Geometry: final body of the model. Coordinates: model frame, mm. Round coordinates to 2 decimals unless told otherwise and drop trailing zeros. Write each loop counter-clockwise with the first axis right and the second up, starting at its lowest first coordinate (ties: lowest second). Pieces come first, ordered by that corner, then holes. Notation, with made-up numbers: (16, 40.5) -> (70, 40.5) arc R33 cw to (70, 74.5) -> close; hole circle Ø6 at (40, 1.25). An arc over 180 degrees is marked (long way). Use one line per item in the form item = value. Start each with the question number.
1. Cut plane B-B, the plane y = -3.5. Return the cut outline in (x, z).
2. Pin query (flat end, axial travel): pin 1 Ø4 at (x, y) = (-7.5, 6.5) entering from -Z; pin 2 Ø9 at (x, y) = (0, 0) entering from -Z; pin 3 Ø2 at (x, y) = (8.5, 12.5) entering from -Z; pin 4 Ø5 at (y, z) = (-4, -10.5) entering from +X. Return the tip coordinate at first contact, or that it passes through.
3. Line query: L1, parallel to Y at x = 0, z = 23.2; L2, parallel to Z at x = -7, y = -2.5; L3, parallel to Z at x = 14.5, y = -9. Output: solid intervals per line, ascending.
4. Cut plane C-C, the plane y = 7. Return the cut outline in (x, z), plus the area to 3 significant figures.
5. Draft query along X for faces 1 (the face through (-4, 3, -23)), 2 (the face through (-5.2, -0.27, -23.43)), 3 (the face through (5.1, -19.5, -22.6)), 4 (the face through (-4, -3, 23)). Return one class per face: pulls with the +X half, pulls with the -X half, needs draft (parallel to the pull), parting line crosses it, or undercut.
6. Cut plane D-D, the plane y = 3. Return the cut outline in (x, z).
7. Cut plane A-A, the plane x = 0. Return the cut outline in (y, z).
Autodesk Inventor part; units mm, degrees
ref_plane "YZ Plane" through (0, 0, 0) normal (1, 0, 0) x (0, 1, 0)
ref_plane "XZ Plane" through (0, 0, 0) normal (0, 1, 0) x (-1, 0, 0)
ref_plane "XY Plane" through (0, 0, 0) normal (0, 0, 1) x (1, 0, 0)
sketch "Эскиз1" plane through (0, 0, 0) normal (0, 0, 1) x (1, 0, 0)
  line L0 (0, 19.5) -> (0, -19.5)
  line L1 (23, -19.5) -> (23, 19.5)
  line L2 (23, 19.5) -> (23.6, 19.5)
  line L3 (24, 19.1) -> (24, -19.1)
  line L4 (23.6, -19.5) -> (23, -19.5)
  line L5 (24, -19.1) -> (23.6, -19.5)
  line L6 (24, 19.1) -> (23.6, 19.5)
  point P0 (0, 0)
  point P1 (0, 0)
  point P2 (24, 19.5)
  point P3 (24, -19.5)
  dimension "d0" = 39
  dimension "d1" = 48
  dimension "d2" = 46
  dimension "d7" = 0.4
  dimension "d8" = 45
  dimension "d9" = 0.4
  dimension "d10" = 45
revolve "Вращение1" add sketch "Эскиз1" angle 360 about axis through (0, 19.5, 0) along (0, -1, 0)
sketch "Эскиз2" plane through (0, 0, 0) normal (0, 0, 1) x (1, 0, 0)
  circle A0 centre (0, 0) radius 5
  dimension "d4" = 10
extrude "Выдавливание1" cut sketch "Эскиз2" along normal through all both and the other way through all
equation "\"d10\" = d8"
properties part number "75. Втулка шестерни третьей передачи"
Outcome:
q1.outline = (-3.57, -23.73) -> (-3.57, -22.72) arc R23 cw to (-3.57, 22.72) -> (-3.57, 23.73) arc R24 ccw to start; (3.57, -23.73) arc R24 ccw to (3.57, 23.73) -> (3.57, 22.72) arc R23 cw to (3.57, -22.72) -> close
q2.pin_1 = -23.36
q2.pin_2 = through
q2.pin_3 = -22.8
q2.pin_4 = 22.63
q3.L1 = -19.5 to -5, 5 to 19.5
q3.L2 = -22.96 to -21.91, 21.91 to 22.96
q3.L3 = -19.12 to -17.85, 17.85 to 19.12
q4.outline = circle Ø48 at (0, 0); hole circle Ø46 at (0, 0)
q4.area = 148 mm^2
q5.face_1 = undercut
q5.face_2 = parting line crosses it
q5.face_3 = needs draft
q5.face_4 = undercut
q6.outline = (-4, -23.66) -> (-4, -22.65) arc R23 cw to (-4, 22.65) -> (-4, 23.66) arc R24 ccw to start; (4, -23.66) arc R24 ccw to (4, 23.66) -> (4, 22.65) arc R23 cw to (4, -22.65) -> close
q7.outline = (-19.5, -23.6) -> (-19.1, -24) -> (-5, -24) -> (-5, -23) -> (-19.5, -23) -> close; (-19.5, 23) -> (-5, 23) -> (-5, 24) -> (-19.1, 24) -> (-19.5, 23.6) -> close; (5, -24) -> (19.1, -24) -> (19.5, -23.6) -> (19.5, -23) -> (5, -23) -> close; (5, 23) -> (19.5, 23) -> (19.5, 23.6) -> (19.1, 24) -> (5, 24) -> close
